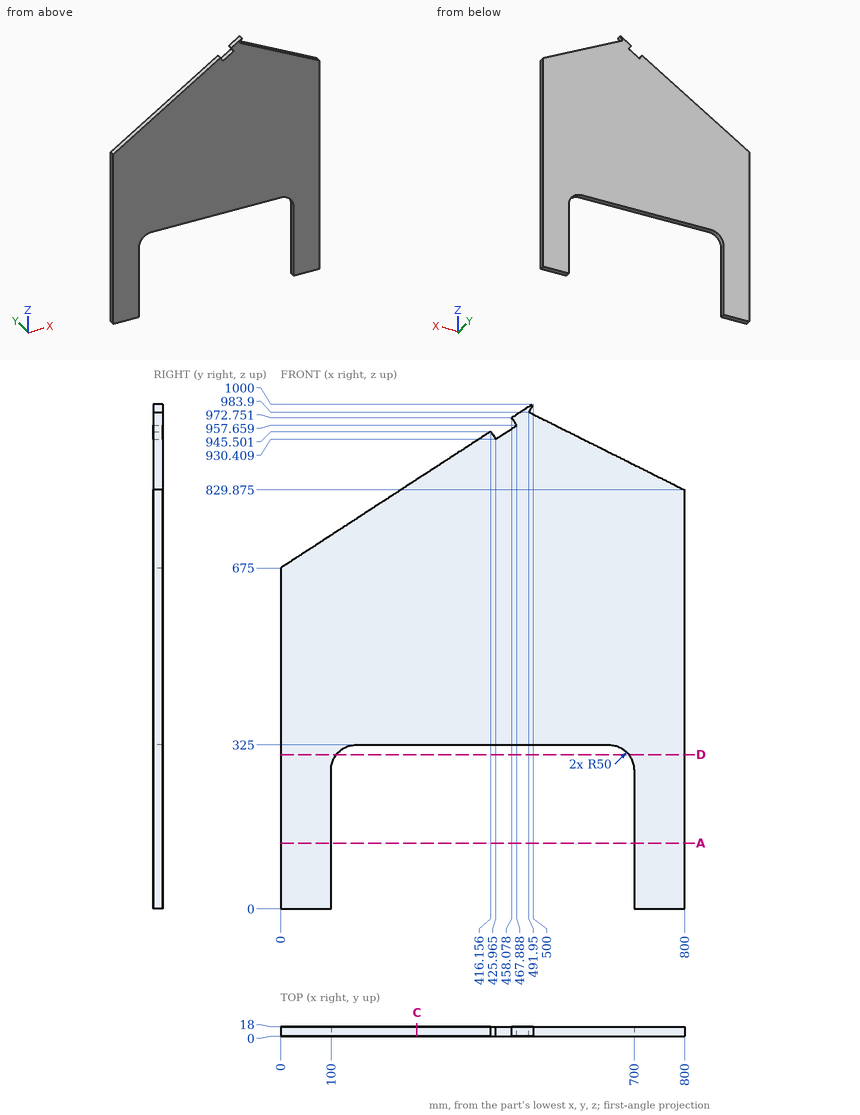
Source: three-view drawing plus pictorial views. Frame: mm from the lowest corner of the part. Round coordinates to 2 decimals unless told otherwise and drop trailing zeros. Write each loop counter-clockwise with the first axis right and the second up, starting at its lowest first coordinate (ties: lowest second). Pieces come first, ordered by that corner, then holes. Notation, with made-up numbers: M -30,49 L -7,49 A12 ccw -7,72 Z; hole C 23.25,32 d10. An arc over 180 degrees is marked long. One line per item, written item: value. Start each with the question number.
Item 1: Section query C-C (x = 270). Return the cut outline in (y, z), plus the area to 3 significant figures.
Item 2: Section query A-A (z = 130.5). Return the cut outline in (x, y).
Item 3: Pin query (flat end, axial travel): pin 1 (8 mm diameter, centred on y = 4, z = 527.5, fed in from -X); pin 2 (10 mm diameter, centred on x = 117.5, y = 7, fed in from -Z); pin 3 (3 mm diameter, centred on y = 9.5, z = 844, fed in from +X); pin 4 (9 mm diameter, centred on x = 395.5, y = 8, fed in from -Z). Return the tip coordinate at first contact, or that it passes through.
Item 4: Ray query, L1, parallel to X at y = 3.5, z = 134; L2, parallel to Z at x = 363.5, y = 17 (1 decimal). Return the intervals inside material, ascending. Write a range as from..to.
Item 5: Section query D-D (z = 305.5). Return the cut outline in (x, y).
Result set:
1. outline: M 0,325 L 18,325 L 18,850.5 L 0,850.5 Z
1. area: 9,460 mm²
2. outline: M 0,0 L 100,0 L 100,18 L 0,18 Z; M 700,0 L 800,0 L 800,18 L 700,18 Z
3. pin 1: stops at x = 0
3. pin 2: stops at z = 308.07
3. pin 3: stops at x = 774.75
3. pin 4: stops at z = 325
4. L1: x = 0..100, 700..800
4. L2: z = 325..911.3
5. outline: M 0,0 L 110.38,0 L 110.38,18 L 0,18 Z; M 689.62,0 L 800,0 L 800,18 L 689.62,18 Z
